Job drawing, mm, ordinate dimensions from the low corner. One solid piece. A direction names the side the tool comes from. Give positions to 0.01 mm unless a question says otherwise; leave off trailing zeros. Write each loop counter-clockwise with the first axis right and the second up, starting at its lowest first coordinate (ties: lowest second). Pieces come first, ordered by that corner, then holes. Notation, with made-up numbers: M 31.5,3.25 L 43.5,3.25 A34 ccw 43.5,40.25 Z; hole C 20.5,-34 d8. An arc over 180 degrees is marked long. Answer as CSV lines item,"result". Start each with the question number.
1) Pin check, flat tip, straight feed: pin 1 Ø5 at (x, y) = (6, 25) entering from -Z. Stop position of the tip, or through.
2) Slice it at A-A, the plane y = 73.58. Give the cut face in (x, z) (3 decimals).
3) Slice it at D-D, the plane x = 5.25. Give the number of separate pieces and of enclosed holes in the cut face, plus the area to 3 significant figures.
4) Slice it at C-C, the plane z = 98.63. Give the cut face in (x, y).
5) Tool access for the marked faces 4, 5 and 6: list every direction of +Z, -Z, +X, -X, +Y, -Y with a clear straight run to the whole face (end or side of a thin tool).
6) Wall check: line 1 along Y through (x, z) = (4.5, 10); line 2 along Z through (x, y) = (6.25, 47); line 3 along Y through (x, z) = (5.75, 78.63). Give the ranges that are in metal, low to high. Write a range as from..to.
7) Slice it at B-B, the plane y = 13.08. Give the cut face in (x, z) (3 decimals), plus the area to 3 significant figures.
8) Mould opens along Y. For the marked faces 1, 2 and 3 say: pulls with the +Y half, pulls with the -Y half, needs draft (parallel to the pull), parting line crosses it, or undercut.
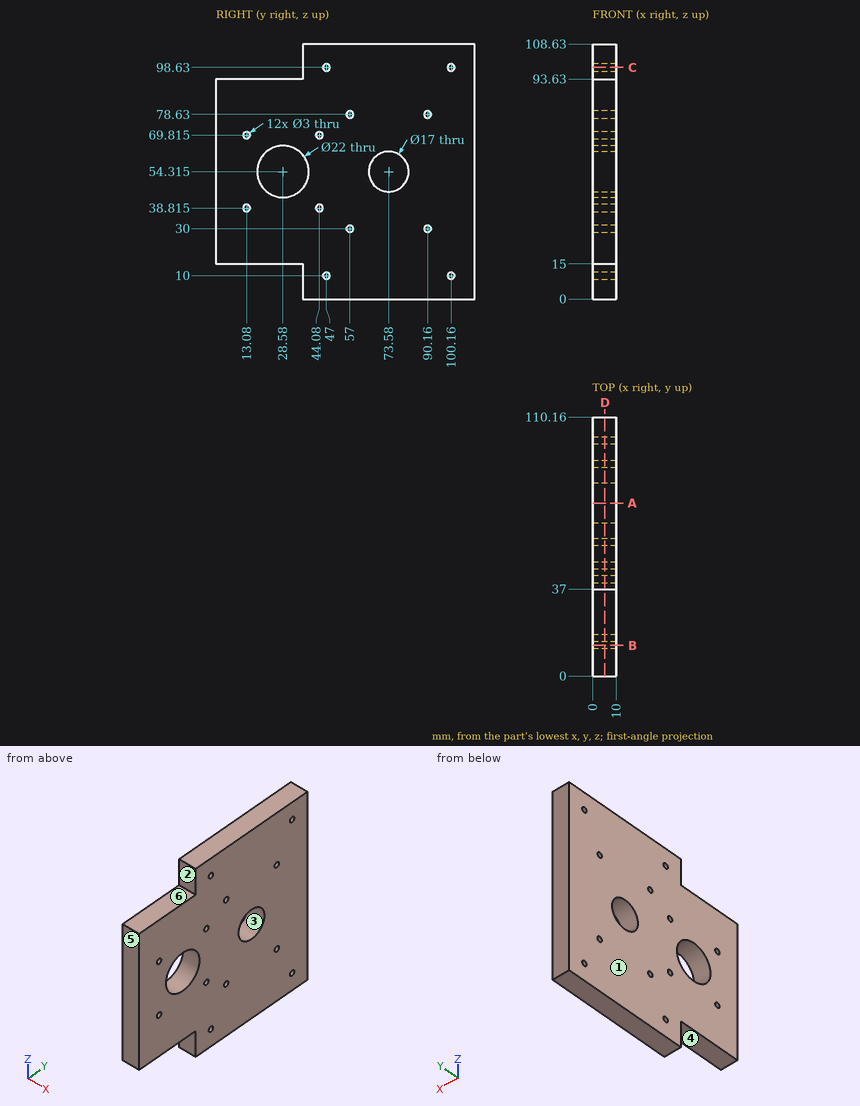
Found:
1,pin 1,"z = 15"
2,outline,"M 0,0 L 10,0 L 10,45.815 L 0,45.815 Z; M 0,62.815 L 10,62.815 L 10,108.63 L 0,108.63 Z"
3,separate pieces,"1"
3,enclosed holes,"14"
3,area,"10,200 mm²"
4,outline,"M 0,37 L 10,37 L 10,45.5 L 0,45.5 Z; M 0,48.5 L 10,48.5 L 10,98.66 L 0,98.66 Z; M 0,101.66 L 10,101.66 L 10,110.16 L 0,110.16 Z"
5,face 4,"-Z, +X, -X, -Y"
5,face 5,"+Z, -Z, +X, -X, -Y"
5,face 6,"+Z, +X, -X, -Y"
6,line 1,"37..45.5, 48.5..98.66, 101.66..110.16"
6,line 2,"0..8.5, 11.5..97.13, 100.13..108.63"
6,line 3,"0..55.5, 58.5..88.66, 91.66..110.16"
7,outline,"M 0,15 L 10,15 L 10,37.315 L 0,37.315 Z; M 0,40.315 L 10,40.315 L 10,68.315 L 0,68.315 Z; M 0,71.315 L 10,71.315 L 10,93.63 L 0,93.63 Z"
7,area,"726 mm²"
8,face 1,"needs draft"
8,face 2,"pulls with the -Y half"
8,face 3,"undercut"
